Could you check a few things on this model? Use its own coordinates, in mm. Face numbers are marked on the shaded views. A direction names the side the tool comes from. Give positions to 0.01 mm unless a question says otherwise; leave off trailing zeros. Order: outer loops, then holes, each group sorted by start corner. A loop starts at its lowest first (then second) coordinate and runs counter-clockwise, first axis right, second up.
(1) Imagine slicing it at A-A, the plane x = 13.5. Write out the boundary of the cut face in (y, z).
(2) Imagine slicing it at C-C, the plane x = 7. Write out the boundary of the cut face in (y, z).
(3) Imagine slicing it at B-B, the plane y = 9.25. Write out the boundary of the cut face in (x, z), then the cut area to 3 significant figures.
(4) If we mould it in two halves opening along Y, with no side actions, what happens to the marked faces 1, 2 and 3? For each: released by +Y, released by -Y, zero draft, split by the parting line, or undercut.
(5) Imagine slicing it at D-D, the plane z = 3. State how many separate pieces and enclosed holes the cut face has, then the cut area to 3 significant figures.
(6) If I drill on probe 1 along X at (y, z) = (1.1, 3); probe 2 along Y at (x, z) = (-11.5, 5); probe 3 along X at (y, z) = (6.5, 4), over which ranges is the centre line in solid material (lowest first)?
(7) On a 3-axis mill with a long thin cutter (end or side, diameter ignored), from which of +Z, -Z, +X, -X, +Y, -Y can I reach the whole of each face in a straight line? I mean the marked faces 4, 5, 6 and 7. Say none if no direction works.
(8) Will these pins go through, and if not, where does the flat tip stop? pin 1 (1.5 mm diameter, centred on y = 7.5, z = 0.5, fed in from +X); pin 2 (0.5 mm diameter, centred on y = 10.5, z = 5.5, fed in from -X); pin 3 (2.5 mm diameter, centred on x = -9, z = 1.5, fed in from +Y).
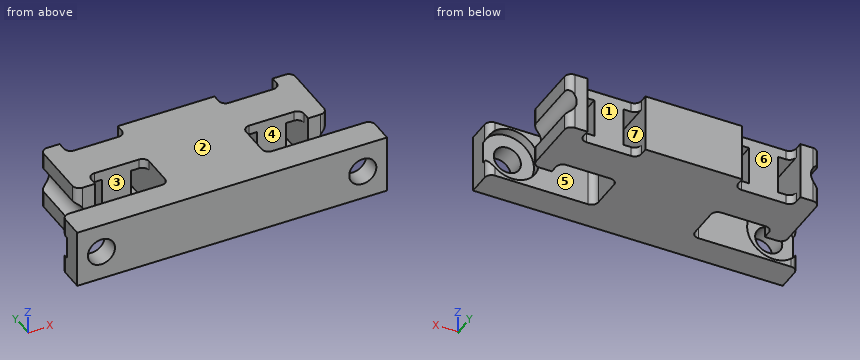
from build123d import *

# Parameters (mm, degrees)
BOSS_EXTRUDE1_DEPTH     = 6
SKETCH4_W               = 6
SKETCH4_H               = 1.5
CUT_EXTRUDE2_DEPTH      = 22.470910554
FILLET1_R               = 0.7
CUT_EXTRUDE1_DEPTH      = 20.798989873
CUT_EXTRUDE1_DEPTH_BACK = 20.798989873
SKETCH2_R               = 1.4
CUT_EXTRUDE3_REACH      = 23.471
SKETCH5_W               = 1.5
SKETCH5_H               = 4
SKETCH6_R               = 2.75
CUT_EXTRUDE5_DEPTH      = 1


with BuildPart() as part:
    # Sketch1 → Boss-Extrude1 (new body)
    with BuildSketch(Plane.XY):
        Polygon((13, 13), (-13, 13), (-13, 6), (-5, 6), (-5, 3), (-16, 3), (-16, 0), (16, 0), (16, 3), (5, 3), (5, 6), (13, 6), align=None)
    extrude(amount=BOSS_EXTRUDE1_DEPTH)

    # Sketch4 → Cut-Extrude2 (cut, through all)
    with BuildSketch(Plane.XY.offset(6)):
        with Locations((-8, 6.75)):
            Rectangle(SKETCH4_W, SKETCH4_H)
        with Locations((-8, 12.25)):
            Rectangle(SKETCH4_W, SKETCH4_H)
        with Locations((8, 12.25)):
            Rectangle(SKETCH4_W, SKETCH4_H)
        with Locations((8, 6.75)):
            Rectangle(SKETCH4_W, SKETCH4_H)
    extrude(amount=-CUT_EXTRUDE2_DEPTH, mode=Mode.SUBTRACT)

    # Fillet1
    fillet1_edges = [part.edges().sort_by_distance(p)[0] for p in [
        (-13, 6, 3),
        (-13, 13, 3),
        (13, 13, 3),
        (13, 6, 3),
        (5, 3, 3),
        (16, 3, 3),
        (-16, 3, 3),
        (-5, 3, 3),
        (5, 7.5, 3),
        (11, 7.5, 3),
        (11, 11.5, 3),
        (5, 11.5, 3),
        (-11, 11.5, 3),
        (-5, 11.5, 3),
        (-11, 7.5, 3),
        (-5, 7.5, 3),
    ]]
    fillet(fillet1_edges, radius=FILLET1_R)

    # Sketch2 → Cut-Extrude1 (cut, two sides: drawn at the far end of the back side and taken through both)
    with BuildSketch(Plane(origin=(0, 3, 0), x_dir=(1, 0, 0), z_dir=(0, 1, 0)).offset(-CUT_EXTRUDE1_DEPTH_BACK)):
        with Locations(Location((-13.5, -3, 0), (0, 0, 180))):
            Circle(SKETCH2_R)
        with Locations(Location((13.5, -3, 0), (0, 0, 180))):
            Circle(SKETCH2_R)
    extrude(amount=CUT_EXTRUDE1_DEPTH + CUT_EXTRUDE1_DEPTH_BACK, mode=Mode.SUBTRACT)

    # Sketch5 → Cut-Extrude3 (cut, up to next)
    with BuildSketch(Plane(origin=(0, 13, 0), x_dir=(1, 0, 0), z_dir=(0, 1, 0)), mode=Mode.PRIVATE) as cut_extrude3_sk1:
        with Locations((-10.25, -3)):
            Rectangle(SKETCH5_W, SKETCH5_H)
    cut_extrude3_tool1 = extrude(cut_extrude3_sk1.sketch, amount=-CUT_EXTRUDE3_REACH, mode=Mode.PRIVATE) & part.part
    # Sketch5 → Cut-Extrude3 (cut, up to next)
    with BuildSketch(Plane(origin=(0, 13, 0), x_dir=(1, 0, 0), z_dir=(0, 1, 0)), mode=Mode.PRIVATE) as cut_extrude3_sk2:
        with Locations((-5.75, -3)):
            Rectangle(SKETCH5_W, SKETCH5_H)
    cut_extrude3_tool2 = extrude(cut_extrude3_sk2.sketch, amount=-CUT_EXTRUDE3_REACH, mode=Mode.PRIVATE) & part.part
    # Sketch5 → Cut-Extrude3 (cut, up to next)
    with BuildSketch(Plane(origin=(0, 13, 0), x_dir=(1, 0, 0), z_dir=(0, 1, 0)), mode=Mode.PRIVATE) as cut_extrude3_sk3:
        with Locations((5.75, -3)):
            Rectangle(SKETCH5_W, SKETCH5_H)
    cut_extrude3_tool3 = extrude(cut_extrude3_sk3.sketch, amount=-CUT_EXTRUDE3_REACH, mode=Mode.PRIVATE) & part.part
    # Sketch5 → Cut-Extrude3 (cut, up to next)
    with BuildSketch(Plane(origin=(0, 13, 0), x_dir=(1, 0, 0), z_dir=(0, 1, 0)), mode=Mode.PRIVATE) as cut_extrude3_sk4:
        with Locations((10.25, -3)):
            Rectangle(SKETCH5_W, SKETCH5_H)
    cut_extrude3_tool4 = extrude(cut_extrude3_sk4.sketch, amount=-CUT_EXTRUDE3_REACH, mode=Mode.PRIVATE) & part.part
    add(cut_extrude3_tool1.solids().sort_by_distance((-10.25, 13, 3))[0], mode=Mode.SUBTRACT)
    add(cut_extrude3_tool2.solids().sort_by_distance((-5.75, 13, 3))[0], mode=Mode.SUBTRACT)
    add(cut_extrude3_tool3.solids().sort_by_distance((5.75, 13, 3))[0], mode=Mode.SUBTRACT)
    add(cut_extrude3_tool4.solids().sort_by_distance((10.25, 13, 3))[0], mode=Mode.SUBTRACT)

    # Sketch6 → Cut-Extrude5 (cut)
    with BuildSketch(Plane(origin=(0, 3, 0), x_dir=(1, 0, 0), z_dir=(0, 1, 0))):
        with Locations((13.5, -3)):
            Circle(SKETCH6_R)
        with Locations((-13.5, -3)):
            Circle(SKETCH6_R)
    extrude(amount=-CUT_EXTRUDE5_DEPTH, mode=Mode.SUBTRACT)


solid = part.part
Answer block:
1. outline: (0, 0) - (3, 0) - (3, 0.25) - (2, 0.25) - (2, 1.6) - (0, 1.6) - close; (0, 4.4) - (2, 4.4) - (2, 5.75) - (3, 5.75) - (3, 6) - (0, 6) - close
2. outline: (0, 0) - (3, 0) - (3, 6) - (0, 6) - close; (7.5, 0) - (11.5, 0) - (11.5, 6) - (7.5, 6) - close
3. outline: (-13, 0) - (13, 0) - (13, 1.69) arc R1.4 cw to (13, 4.31) - (13, 6) - (-13, 6) - (-13, 4.31) arc R1.4 cw to (-13, 1.69) - close; hole (-11, 1) - (-9.5, 1) - (-9.5, 5) - (-11, 5) - close; hole (-6.5, 1) - (-5, 1) - (-5, 5) - (-6.5, 5) - close; hole (5, 1) - (6.5, 1) - (6.5, 5) - (5, 5) - close; hole (9.5, 1) - (11, 1) - (11, 5) - (9.5, 5) - close
3. area: 129 mm2
4. face 1: released by +Y
4. face 2: zero draft
4. face 3: undercut
5. separate pieces: 7
5. enclosed holes: 0
5. area: 214 mm2
6. probe 1: x = -16 to -14.9, -12.1 to 12.1, 14.9 to 16
6. probe 2: y = 0 to 3, 6 to 13
6. probe 3: x = -12.52 to -11, -5 to 5, 11 to 12.52
7. face 4: +Z, -Z
7. face 5: +Z, -Z, +X
7. face 6: +Z, -Z, +Y
7. face 7: none
8. pin 1: stops at x = 13
8. pin 2: stops at x = -13
8. pin 3: stops at y = 11.5
